Can you work these out from the drawing? Everything is in mm from the part's minimum corner. A direction names the side the tool comes from. Give positions to 0.01 mm unless a question says otherwise; leave off trailing zeros. Loops run counter-clockwise (first coordinate to the right, second up) from the corner with the lowest first, then second, coordinate; pieces in that order, holes last. Notation, with made-up numbers: (55, 67.5) - (88, 67.5) arc R19 cw to (88, 101.5) - close; hole circle Ø8 at (-19, 53.5). An arc over 180 degrees is marked (long way). Answer in a Markdown table with one row per item. Add a question column.
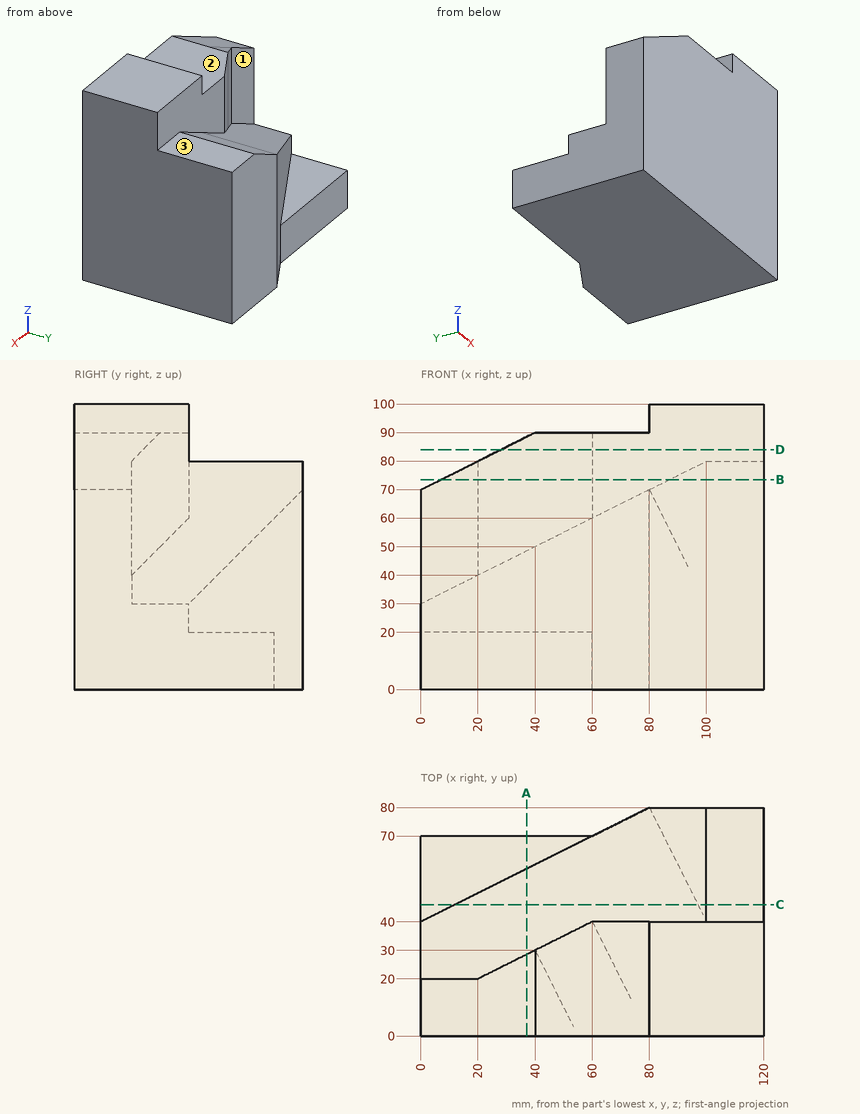
(1) Please list where these lines run through material, in increasing order: line 1 (Y direction, x = 79, z = 83); line 2 (Z direction, x = 60, y = 64); line 3 (Y direction, x = 46, z = 10.5).
(2) I want a section at D-D on z = 84. Please give me the cut outline in (x, y).
(3) I want a section at C-C on y = 46. Please give me the cut outline in (x, z), then the cut area to 3 significant figures.
(4) I want a section at A-A on x = 37. Please give me the cut outline in (y, z), then the cut area to 3 significant figures.
(5) I want a section at B-B on z = 73.5. Please give me the cut outline in (x, y).
(6) On a 3-axis mill with a long thin cutter (end or side, diameter ignored), from which of +Z, -Z, +X, -X, +Y, -Y can I reach the whole of each face in a straight line? I mean the marked faces 1, 2 and 3. Say none if no direction works.
(7) For pin 1 Ø12 at (x, y) = (70, 14) entering from +Z; pin 2 Ø1 at (y, z) = (23.5, 76) entering from -X; pin 3 Ø4 at (y, z) = (37, 67) entering from -X, each with a flat end and sliding along its axis, tell me the tip position at first contact or that it passes through.
Reported:
| question | item | result |
|---|---|---|
| 1 | line 1 | 0 to 40 |
| 1 | line 2 | 0 to 60 |
| 1 | line 3 | 0 to 70 |
| 2 | outline | (28, 0) - (120, 0) - (120, 40) - (60, 40) - (28, 24) - close |
| 3 | outline | (0, 0) - (120, 0) - (120, 80) - (100, 80) - (12, 36) - (12, 20) - (0, 20) - close |
| 3 | area | 6,940 mm² |
| 4 | outline | (0, 0) - (70, 0) - (70, 20) - (58.5, 20) - (58.5, 48.5) - (28.5, 48.5) - (28.5, 88.5) - (0, 88.5) - close |
| 4 | area | 4,210 mm² |
| 5 | outline | (7, 0) - (120, 0) - (120, 80) - (87, 80) - (87, 40) - (60, 40) - (20, 20) - (7, 20) - close |
| 6 | face 1 | +Z, -X, +Y |
| 6 | face 2 | +Z, -X, +Y, -Y |
| 6 | face 3 | +Z, +X, -X, +Y |
| 7 | pin 1 | z = 90 |
| 7 | pin 2 | x = 26 |
| 7 | pin 3 | x = 50 |
